Model file for the job. Use its own axes, mm. A direction names the side the tool comes from. Give positions to 0.01 mm unless a question says otherwise; leave off trailing zeros. Order: outer loops, then holes, each group sorted by start corner. A loop starts at its lowest first (then second) coordinate and runs counter-clockwise, first axis right, second up. Notation, with made-up numbers: (66.5, 82) -> (85.5, 82) arc R21 ccw to (85.5, 88) -> close; hole circle Ø8 at (-17.75, 19). An arc over 180 degrees is marked (long way). Answer in a Markdown table with one row per item. Add a question column.
from build123d import *

# Parameters (mm, degrees)
EXTRUDE_1_DEPTH     = 2.5
EXTRUDE_START       = -2.5
EXTRUDE_2_DEPTH     = 5
EXTRUDE_4_DEPTH     = 4
SKETCH_9_W          = 5
SKETCH_9_H          = 5
CUT_EXTRUDE_4_DEPTH = 8
SKETCH_10_W         = 5
SKETCH_10_H         = 12.173237657
EXTRUDE_5_DEPTH     = 10
CHAMFER_2_SIZE      = 1
CHAMFER_3_SIZE      = 1


with BuildPart() as part:
    # 草图1 → 凸台-拉伸1 (new body, symmetric)
    with BuildSketch(Plane(origin=(0, 0, 0), x_dir=(0, 0, -1), z_dir=(1, 0, 0))):
        with BuildLine():
            ThreePointArc((-12.012209006, 35.102143532), (-13.602346238, 34.762025687), (-15.159597133, 34.293852416))
            Line((-15.159597133, 34.293852416), (-14.475556847, 36.173237657))
            Line((-14.475556847, 36.173237657), (0, 36.173237657))
            Line((0, 36.173237657), (4, 36.173237657))
            Line((4, 36.173237657), (4, 0))
            Line((4, 0), (0, 0))
            Line((0, 0), (0, 13.821800738))
            Line((0, 13.821800738), (-2, 15.5))
            Line((-2, 15.5), (0, 15.5))
            ThreePointArc((0, 15.5), (-1.024954416, 16.762412377), (-2.149076967, 17.937386868))
            Line((-2.149076967, 17.937386868), (-0.163984664, 18.181125555))
            ThreePointArc((-0.163984664, 18.181125555), (-1.335148592, 19.30921758), (-2.594085474, 20.338437912))
            Line((-2.594085474, 20.338437912), (-0.653494022, 20.822281703))
            ThreePointArc((-0.653494022, 20.822281703), (-1.953408107, 21.799236122), (-3.32839147, 22.667358991))
            Line((-3.32839147, 22.667358991), (-1.461230617, 23.38409489))
            ThreePointArc((-1.461230617, 23.38409489), (-2.870516133, 24.195347563), (-4.341048143, 24.889431256))
            Line((-4.341048143, 24.889431256), (-2.575152957, 25.828374381))
            ThreePointArc((-2.575152957, 25.828374381), (-4.072800703, 26.4618314), (-5.616959114, 26.971528727))
            Line((-5.616959114, 26.971528727), (-3.978655026, 28.1186816))
            ThreePointArc((-3.978655026, 28.1186816), (-5.542338523, 28.564899578), (-7.13710349, 28.882612127))
            Line((-7.13710349, 28.882612127), (-5.65081384, 30.22087334))
            ThreePointArc((-5.65081384, 30.22087334), (-7.257222169, 30.473200196), (-8.87881942, 30.594191604))
            Line((-8.87881942, 30.594191604), (-7.566701362, 32.103610765))
            ThreePointArc((-7.566701362, 32.103610765), (-9.191886676, 32.158284886), (-10.816141931, 32.080751451))
            Line((-10.816141931, 32.080751451), (-9.697756124, 33.738826596))
            ThreePointArc((-9.697756124, 33.738826596), (-11.317490652, 33.595032918), (-12.920190005, 33.320130484))
            Line((-12.920190005, 33.320130484), (-12.012209006, 35.102143532))
        make_face()
    extrude(amount=EXTRUDE_1_DEPTH, both=True)

    # 草图6 → 凸台-拉伸2 (add)
    with BuildSketch(Plane(origin=(0, 0, 0), x_dir=(0, 0, -1), z_dir=(1, 0, 0)).offset(EXTRUDE_START)):
        Polygon((14.9, 31.95), (11, 31.95), (9, 29.95), (5, 29.95), (4, 30.95), (4, 7.05), (5, 8.05), (9, 8.05), (11, 6.05), (14.9, 6.05), align=None)
    extrude(amount=EXTRUDE_2_DEPTH)

    # 草图8 → 凸台-拉伸4 (add)
    with BuildSketch(Plane.XY):
        Polygon((-2.5, 0), (-3.9, 0), (-3.9, 1.9), (-2.5, 4.324871131), align=None)
    extrude(amount=-EXTRUDE_4_DEPTH)

    # 草图9 → 切除-拉伸4 (cut)
    with BuildSketch(Plane(origin=(0, 0, -14.9), x_dir=(-1, 0, 0), z_dir=(0, 0, -1))):
        with Locations((0, 24)):
            Rectangle(SKETCH_9_W, SKETCH_9_H)
    extrude(amount=-CUT_EXTRUDE_4_DEPTH, mode=Mode.SUBTRACT)

    # 草图10 → 凸台-拉伸5 (add)
    with BuildSketch(Plane(origin=(0, 0, 0), x_dir=(0, 0, -1), z_dir=(1, 0, 0))):
        with Locations((1.5, 30.086618829)):
            Rectangle(SKETCH_10_W, SKETCH_10_H)
    extrude(amount=-EXTRUDE_5_DEPTH)

    # 倒角2
    chamfer_2_edges = [part.edges().sort_by_distance(p)[0] for p in [
        (0, 26.5, -14.9),
        (0, 21.5, -6.9),
        (0, 26.5, -6.9),
        (0, 21.5, -14.9),
        (0, 6.05, -14.9),
        (0, 31.95, -14.9),
    ]]
    chamfer(chamfer_2_edges, length=CHAMFER_2_SIZE)

    # 倒角3
    chamfer_3_edges = [part.edges().sort_by_distance(p)[0] for p in [
        (-2.5, 30.086618829, 1),
        (-2.5, 27.475, -4),
    ]]
    chamfer(chamfer_3_edges, length=CHAMFER_3_SIZE)


solid = part.part
Item 1: Pin check, flat tips, straight feed: pin 1 Ø0.9 at (x, y) = (-0.5, 24.5) entering from -Z; pin 2 Ø4 at (x, z) = (-3.5, 8.5) entering from -Y; pin 3 Ø3 at (x, y) = (-7.5, 32) entering from +Z. Stop position of each tip, or through.
Item 2: Saw through at C-C on y = 5.5. List the corners of the cut face in (x, z), plus the area to 3 significant figures.
Item 3: Wall check: line 1 (Y direction, x = -0.5, z = -8.5); line 2 (X direction, y = 22, z = 0); line 3 (Y direction, x = -6.25, z = -2). Give the ranges that are in metal, low to high.
Item 4: Two-plate mould, pull along Y, no slides. Class faces 4 (the flat face through (2.5, 18, -3)), 5 (the cylindrical face through (0.035, 21.786, 1.935)), 6 (the flat face through (0, 6.05, -12)), 7 (the flat face through (0, 29.95, -7)): pulls with the +Y half, pulls with the -Y half, needs draft (parallel to the pull), parting line crosses it, or undercut.
Item 5: Saw through at A-A on z = -10.5. List the corners of the cut face in (x, y).
Item 6: Which spindle directions (+Z, -Z, +X, -X, +Y, -Y) get a long thin tool onto all of the face, cutting with end or side? Do faces 1 (the flat face through (0, 21.5, -11)), 2 (the flat face through (-0.04, 7.54, -4.49)), 3 (the flat face through (-1, 36.173, 3)). Say none if no direction does.
Item 7: Saw through at B-B on x = -6.25. List the corners of the cut face in (y, z).
Evaluation:
| question | item | result |
|---|---|---|
| 1 | pin 1 | stops at z = -6.9 |
| 1 | pin 2 | stops at y = 28.82 |
| 1 | pin 3 | stops at z = 1 |
| 2 | outline | (-2.5, -4) -> (2.5, -4) -> (2.5, 0) -> (-2.5, 0) -> close |
| 2 | area | 20.0 mm2 |
| 3 | line 1 | y = 8.05 to 21.5, 26.5 to 29.95 |
| 3 | line 2 | x = -2.5 to 2.5 |
| 3 | line 3 | y = 24 to 36.17 |
| 4 | face 4 | needs draft |
| 4 | face 5 | undercut |
| 4 | face 6 | pulls with the -Y half |
| 4 | face 7 | pulls with the +Y half |
| 5 | outline | (-2.5, 6.55) -> (2.5, 6.55) -> (2.5, 21.5) -> (-2.5, 21.5) -> close; (-2.5, 26.5) -> (2.5, 26.5) -> (2.5, 31.45) -> (-2.5, 31.45) -> close |
| 6 | face 1 | -Z, +X, -X |
| 6 | face 2 | +X, -X, -Y |
| 6 | face 3 | +Z, -Z, +X, -X, +Y |
| 7 | outline | (24, -4) -> (36.17, -4) -> (36.17, 1) -> (24, 1) -> close |
